```python
from build123d import *

# Parameters (mm, degrees)
SKETCH1_R           = 0.5
BOSS_EXTRUDE1_DEPTH = 3.333333
SKETCH2_R           = 2
BOSS_EXTRUDE2_DEPTH = 16
SCALE1_SCALE        = 2.5


with BuildPart() as part:
    # Sketch1 → Boss-Extrude1 (new body)
    with BuildSketch(Plane(origin=(0, 0, 0), x_dir=(1, 0, 0), z_dir=(0, 1, 0))):
        with Locations(Location((0, 0, 0), (0, 0, 270))):
            Circle(SKETCH1_R)
    extrude(amount=-BOSS_EXTRUDE1_DEPTH)

    # Sketch2 → Boss-Extrude2 (add)
    with BuildSketch(Plane.XZ.offset(3.333333)):
        with Locations(Location((0, 0, 0), (0, 0, 270))):
            Circle(SKETCH2_R)
    extrude(amount=BOSS_EXTRUDE2_DEPTH)


with BuildPart() as part_1:
    # Scale1: scaled about (0, -11.2090828, 0)
    add(part.part.scale(SCALE1_SCALE).moved(Location((0, 16.8136242, 0))))


solid = part_1.part
```
Verification items for the finished model (mm, model axes). A direction names the side the tool comes from. Coordinates: 2 decimals unless noted, no trailing zeros. Order: outer loops, then holes, each group sorted by start corner. A loop starts at its lowest first (then second) coordinate and runs counter-clockwise, first axis right, second up. Notation, with made-up numbers: (-39, 38) - (-29, 38) arc R9 ccw to (-29, 55) - close; hole circle Ø1 at (85.25, 16.25). An arc over 180 degrees is marked (long way). Return JSON: item names as keys, results as strings.
(1) Section check C-C, the plane y = 7. Record the cut outline in (x, z), and give its area (3 significant figures).
Filled sheet:
{"outline": "circle Ø10 at (0, 0)", "area": "78.5 mm^2"}
(2) Thickness scan on line 1 along Y through (x, z) = (-4, 1.25); line 2 along X through (y, z) = (-22, -0.25). Record the ranges inside material, lowest first.
Filled sheet:
{"line 1": "y = -31.52 to 8.48", "line 2": "x = -4.99 to 4.99"}
(3) Section check D-D, the plane z = -3. Record the cut outline in (x, y).
Filled sheet:
{"outline": "(-4, -31.52) - (4, -31.52) - (4, 8.48) - (-4, 8.48) - close"}
(4) Go/stop test with a flat-tipped pin: pin 1 (1.5 mm diameter, centred on y = 6, z = -1, fed in from +X). Record where the tip stops, or that it passes through.
Filled sheet:
{"pin 1": "stops at x = 4.99"}
(5) Access from +Z, -Z, +X, -X, +Y, -Y to the whole of each face (thin tool, end or side, straight path). Record for faces 1 (the flat face through (0, -31.52, 0)), 2 (the cylindrical face through (-1.22, 12.71, -0.27)).
Filled sheet:
{"face 1": "+Z, -Z, +X, -X, -Y", "face 2": "+Y"}
(6) Section check A-A, the plane x = 0. Record the cut outline in (y, z), and give its area (3 significant figures).
Filled sheet:
{"outline": "(-31.52, -5) - (8.48, -5) - (8.48, -1.25) - (16.81, -1.25) - (16.81, 1.25) - (8.48, 1.25) - (8.48, 5) - (-31.52, 5) - close", "area": "421 mm^2"}
(7) Section check B-B, the plane z = 0. Record the cut outline in (x, y).
Filled sheet:
{"outline": "(-5, -31.52) - (5, -31.52) - (5, 8.48) - (1.25, 8.48) - (1.25, 16.81) - (-1.25, 16.81) - (-1.25, 8.48) - (-5, 8.48) - close"}
